```python
from build123d import *

# Parameters (mm, degrees)
SKETCH1_R                      = 45
BOSS_EXTRUDE1_DEPTH            = 20
SKETCH2_R                      = 30
BOSS_EXTRUDE2_DEPTH            = 160
SKETCH3_R                      = 45
BOSS_EXTRUDE3_DEPTH            = 20
SKETCH4_R                      = 12.5
BOSS_EXTRUDE4_DEPTH            = 5
M8X1_25_TAPPED_HOLE1_REACH     = 202
M8X1_25_TAPPED_HOLE1_BORE_R    = 3.4
CIRPATTERN1_COUNT              = 6
F_8_5_8_5_DIAMETER_HOLE1_D     = 8.5
F_8_5_8_5_DIAMETER_HOLE1_DEPTH = 20.001
CIRPATTERN2_COUNT              = 6
SKETCH11_R                     = 12.5
CUT_EXTRUDE1_DEPTH             = 20


with BuildPart() as part:
    # Sketch1 → Boss-Extrude1 (new body)
    with BuildSketch(Plane.XY):
        Circle(SKETCH1_R)
    extrude(amount=BOSS_EXTRUDE1_DEPTH)

    # Sketch2 → Boss-Extrude2 (add)
    with BuildSketch(Plane(origin=(0, 0, 0), x_dir=(-1, 0, 0), z_dir=(0, 0, -1))):
        Circle(SKETCH2_R)
    extrude(amount=BOSS_EXTRUDE2_DEPTH)

    # Sketch3 → Boss-Extrude3 (add)
    with BuildSketch(Plane(origin=(0, 0, -160), x_dir=(-1, 0, 0), z_dir=(0, 0, -1))):
        with Locations(Location((0, 0, 0), (0, 0, 180))):  # turned: the seam where the file's is
            Circle(SKETCH3_R)
    extrude(amount=BOSS_EXTRUDE3_DEPTH)

    # Sketch4 → Boss-Extrude4 (add)
    with BuildSketch(Plane.XY.offset(20)):
        Circle(SKETCH4_R)
    extrude(amount=BOSS_EXTRUDE4_DEPTH)

    # M8x1.25 Tapped Hole1 bore → M8x1.25 Tapped Hole1 (cut, up to next)
    with BuildSketch(Plane.XY.offset(20), mode=Mode.PRIVATE) as m8x1_25_tapped_hole1_sk1:
        with Locations((0, 37.5)):
            Circle(M8X1_25_TAPPED_HOLE1_BORE_R)
    m8x1_25_tapped_hole1_tool1 = extrude(m8x1_25_tapped_hole1_sk1.sketch, amount=-M8X1_25_TAPPED_HOLE1_REACH, mode=Mode.PRIVATE) & part.part
    m8x1_25_tapped_hole1 = m8x1_25_tapped_hole1_tool1.solids().sort_by_distance((0, 37.5, 20))[0]
    add(m8x1_25_tapped_hole1, mode=Mode.SUBTRACT)

    # CirPattern1: M8x1.25 Tapped Hole1 ×6 about axis
    cirpattern1_axis = Axis((0, 0, 0), (0, 0, 1))
    for i in range(1, CIRPATTERN1_COUNT):
        add(m8x1_25_tapped_hole1.rotate(cirpattern1_axis, i * 360 / CIRPATTERN1_COUNT), mode=Mode.SUBTRACT)

    # Ø8.5 (8.5) Diameter Hole1
    with Locations(Plane(origin=(0, 0, -180), x_dir=(-1, 0, 0), z_dir=(0, 0, -1))):
        with Locations((0, 37.5)):
            f_8_5_8_5_diameter_hole1 = Hole(F_8_5_8_5_DIAMETER_HOLE1_D / 2, depth=F_8_5_8_5_DIAMETER_HOLE1_DEPTH)

    # CirPattern2: Ø8.5 (8.5) Diameter Hole1 ×6 about axis
    cirpattern2_axis = Axis((0, 0, 0), (0, 0, 1))
    for i in range(1, CIRPATTERN2_COUNT):
        add(f_8_5_8_5_diameter_hole1.rotate(cirpattern2_axis, i * 360 / CIRPATTERN2_COUNT), mode=Mode.SUBTRACT)

    # Sketch11 → Cut-Extrude1 (cut)
    with BuildSketch(Plane(origin=(0, 0, -180), x_dir=(-1, 0, 0), z_dir=(0, 0, -1))):
        with Locations(Location((0, 0, 0), (0, 0, 180))):  # turned: the seam where the file's is
            Circle(SKETCH11_R)
    extrude(amount=-CUT_EXTRUDE1_DEPTH, mode=Mode.SUBTRACT)


solid = part.part
```
Geometry check sheet. Reference: the model listing, model coordinates, mm. A direction names the side the tool comes from. Give positions to 0.01 mm unless a question says otherwise; leave off trailing zeros. Order: outer loops, then holes, each group sorted by start corner. A loop starts at its lowest first (then second) coordinate and runs counter-clockwise, first axis right, second up. Notation, with made-up numbers: (50, -39) - (55, -39) arc R28 cw to (55, -19) - close; hole circle Ø8 at (16, -27). An arc over 180 degrees is marked (long way). Answer in a Markdown table with one row per item. Add a question column.
Q1. Tool access check on faces 1 (the flat face through (9, 9, -180)), 2 (the cylindrical face through (29.08, -18.6, 10.14)), 3 (the flat face through (9, -9, 20)), 4 (the flat face through (9, 29, -160)), 5 (the cylindrical face through (-29.34, 15.88, -169.86)). Record the directions out of +Z, -Z, +X, -X, +Y, -Y that give a thin tool (end or side, any length) a straight path to the whole face; none if there is none.
Q2. Cross-section at C-C, the plane y = 27.5. Enter the section's corners in (x, z), then the cut area to 3 significant figures.
Q3. Mould release check, pull along X, two halves, no side actions. Record for faces 6 (the cylindrical face through (-0.44, 40.87, 10.14)), 7 (the cylindrical face through (20.765, 39.923, -169.86)), 8 (the flat face through (29, -9, 0)): pulls with the +X half, pulls with the -X half, needs draft (parallel to the pull), parting line crosses it, or undercut.
Q4. Cross-section at A-A, the plane y = -37.5. Enter the section's corners in (x, z), then the cut area to 3 significant figures.
Q5. Material ranges on probe 1 along Y at (x, z) = (0, -166.25); probe 2 along Y at (x, z) = (0, 5); probe 3 along Z at (x, y) = (-12, 18), recorded low to high. Write a range as from..to.
Q6. Cross-section at D-D, the plane x = 0. Count the separate pieces of the cut face and the enclosed holes in it, then the cut area to 3 significant figures.
Q7. Cross-section at B-B, the plane x = 17. Enter the section's corners in (y, z).
Q8. Gauge pin test, flat ends, axial feed: pin 1 (5 mm diameter, centred on y = -33.5, z = -62.5, fed in from -X); pin 2 (6 mm diameter, centred on y = 21, z = -145.5, fed in from +X); pin 3 (1 mm diameter, centred on x = 18, z = -4, fed in from +Y); pin 4 (4 mm diameter, centred on y = -27.5, z = -24, fed in from -X). Record the tip position at first contact, or that the pin passes through.
Check values:
| question | item | result |
|---|---|---|
| 1 | face 1 | -Z, +X, -X, +Y, -Y |
| 1 | face 2 | +Z, -Z |
| 1 | face 3 | +Z |
| 1 | face 4 | none |
| 1 | face 5 | -Z |
| 2 | outline | (-35.62, -180) - (35.62, -180) - (35.62, -160) - (11.99, -160) - (11.99, 0) - (35.62, 0) - (35.62, 20) - (-35.62, 20) - (-35.62, 0) - (-11.99, 0) - (-11.99, -160) - (-35.62, -160) - close |
| 2 | area | 6,690 mm^2 |
| 3 | face 6 | undercut |
| 3 | face 7 | parting line crosses it |
| 3 | face 8 | needs draft |
| 4 | outline | (-24.87, -180) - (-4.25, -180) - (-4.25, -160) - (-24.87, -160) - close; (-24.87, 0) - (-3.4, 0) - (-3.4, 20) - (-24.87, 20) - close; (3.4, 0) - (24.87, 0) - (24.87, 20) - (3.4, 20) - close; (4.25, -180) - (24.87, -180) - (24.87, -160) - (4.25, -160) - close |
| 4 | area | 1,680 mm^2 |
| 5 | probe 1 | y = -45..-41.75, -33.25..-12.5, 12.5..33.25, 41.75..45 |
| 5 | probe 2 | y = -45..-40.9, -34.1..34.1, 40.9..45 |
| 5 | probe 3 | z = -180..20 |
| 6 | separate pieces | 5 |
| 6 | enclosed holes | 0 |
| 6 | area | 12,200 mm^2 |
| 7 | outline | (-41.67, -180) - (41.67, -180) - (41.67, -160) - (24.72, -160) - (24.72, 0) - (41.67, 0) - (41.67, 20) - (-41.67, 20) - (-41.67, 0) - (-24.72, 0) - (-24.72, -160) - (-41.67, -160) - close |
| 8 | pin 1 | passes through |
| 8 | pin 2 | stops at x = 24 |
| 8 | pin 3 | stops at y = 24.37 |
| 8 | pin 4 | stops at x = -15.8 |
